Here's the drawing with two shaded views (mm, measured from the low corner). I have some questions. Coordinates: 2 decimals unless noted, no trailing zeros. Write each loop counter-clockwise with the first axis right and the second up, starting at its lowest first coordinate (ties: lowest second). Pieces come first, ordered by that corner, then holes. Notation, with made-up numbers: (17.25, -35.75) - (43.25, -35.75) arc R16 ccw to (43.25, -7.75) - close; hole circle Ø2 at (-2.5, 82.25). An arc over 180 degrees is marked (long way). Answer in a Markdown table with one row per item. Add a question column.
Item 1: If I drill on probe 1 along Y at (x, z) = (98, 2.35); probe 2 along X at (y, z) = (165, 2.7); probe 3 along X at (y, z) = (144, 1.6), over which ranges is the centre line in solid material (lowest first)? Write a range as from..to.
Item 2: Imagine slicing it at D-D (x = 56). Please give me the cut outline in (y, z).
Item 3: Imagine slicing it at A-A (x = 85). Please give me the cut outline in (y, z), plus the area to 3 significant figures.
Item 4: Imagine slicing it at C-C (z = 2.95). State how many separate pieces and enclosed holes the cut face has, plus the area to 3 significant figures.
Item 5: Imagine slicing it at B-B (y = 112). Please give me the cut outline in (x, z), plus the area to 3 significant figures.
Item 6: I'm going to push flat-ended pins straight in: pin 1 (3 mm diameter, centred on x = 58.5, z = 1, fed in from -Y); pin 2 (1.5 mm diameter, centred on y = 228.5, z = 1.5, fed in from +X); pin 3 (2.5 mm diameter, centred on x = 18, z = 3, fed in from -Y). Where does each tip first touch, or does it pass through?
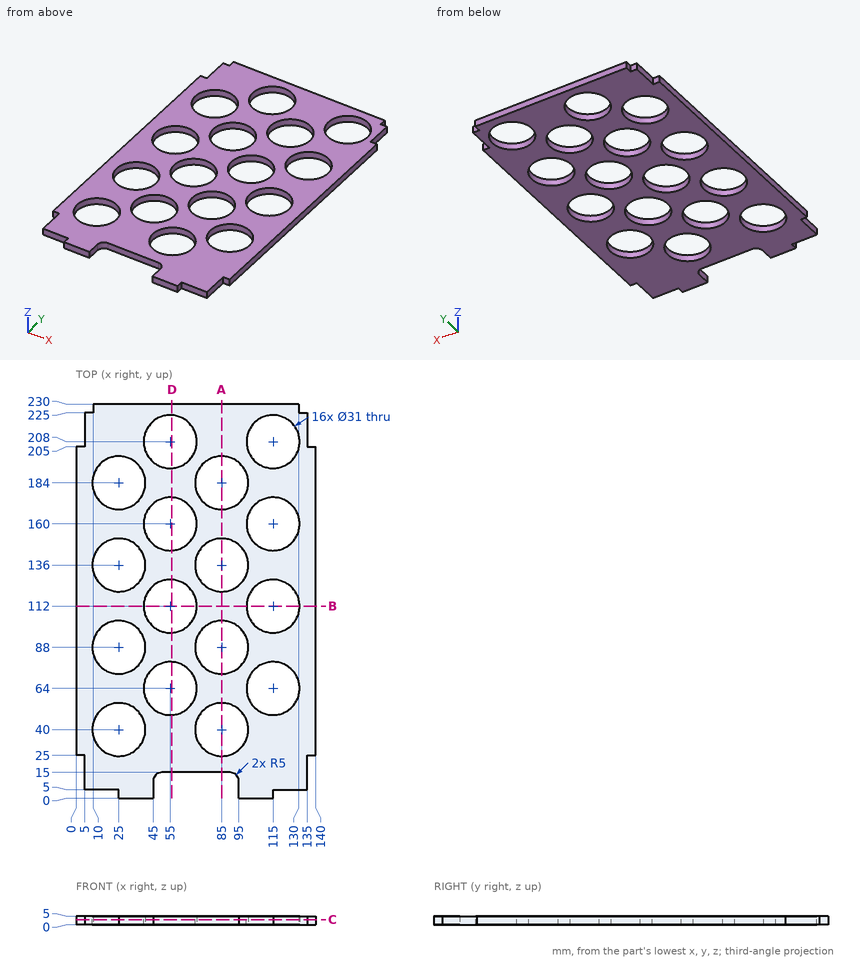
Here are the results:
| question | item | result |
|---|---|---|
| 1 | probe 1 | y = 0..31.56, 48.44..79.56, 96.44..127.56, 144.44..175.56, 192.44..230 |
| 1 | probe 2 | x = 0..40.33, 69.67..100.33, 129.67..140 |
| 1 | probe 3 | x = 0..11.72, 38.28..71.72, 98.28..140 |
| 2 | outline | (15, 0) - (48.53, 0) - (48.53, 5) - (15, 5) - close; (79.47, 0) - (96.53, 0) - (96.53, 5) - (79.47, 5) - close; (127.47, 0) - (144.53, 0) - (144.53, 5) - (127.47, 5) - close; (175.47, 0) - (192.53, 0) - (192.53, 5) - (175.47, 5) - close; (223.47, 0) - (230, 0) - (230, 5) - (223.47, 5) - close |
| 3 | outline | (15, 0) - (24.5, 0) - (24.5, 5) - (15, 5) - close; (55.5, 0) - (72.5, 0) - (72.5, 5) - (55.5, 5) - close; (103.5, 0) - (120.5, 0) - (120.5, 5) - (103.5, 5) - close; (151.5, 0) - (168.5, 0) - (168.5, 5) - (151.5, 5) - close; (199.5, 0) - (230, 0) - (230, 5) - (199.5, 5) - close |
| 3 | area | 455 mm2 |
| 4 | separate pieces | 1 |
| 4 | enclosed holes | 16 |
| 4 | area | 18,600 mm2 |
| 5 | outline | (0, 0) - (39.5, 0) - (39.5, 5) - (0, 5) - close; (70.5, 0) - (99.5, 0) - (99.5, 5) - (70.5, 5) - close; (130.5, 0) - (140, 0) - (140, 5) - (130.5, 5) - close |
| 5 | area | 390 mm2 |
| 6 | pin 1 | stops at y = 15 |
| 6 | pin 2 | stops at x = 130 |
| 6 | pin 3 | stops at y = 5 |
